Read the model definition and answer for the solid it produces. Units are mm, in the model's axes. A direction names the side the tool comes from. Coordinates: 2 decimals unless noted, no trailing zeros. Write each loop counter-clockwise with the first axis right and the second up, starting at its lowest first coordinate (ties: lowest second). Pieces come first, ordered by that corner, then holes. Notation, with made-up numbers: (33, 2.25) -> (56, 2.25) arc R14 ccw to (56, 20.25) -> close; hole circle Ø2 at (73.25, 89). An arc over 180 degrees is marked (long way). Return JSON: item names as keys, results as strings.
from build123d import *

# Parameters (mm, degrees)
BOSS_EXTRUDE1_DEPTH = 3.81
SKETCH3_R           = 2.3749
BOSS_EXTRUDE2_DEPTH = 8.89


with BuildPart() as part:
    # Sketch1 → Boss-Extrude1 (new body)
    with BuildSketch(Plane(origin=(0, 0, 0), x_dir=(-1, 0, 0), z_dir=(0, 0, 1))):
        with BuildLine():
            Line((22.628547269, -66.432139719), (24.16561852, -64.81086345))
            ThreePointArc((24.16561852, -64.81086345), (34.487993287, -48.673067402), (38.1, -29.859952573))
            Line((38.1, -29.859952573), (38.1, -15.158740079))
            Line((38.1, -15.158740079), (19.05, -15.158740079))
            Line((19.05, -15.158740079), (19.05, -38.1))
            ThreePointArc((19.05, -38.1), (15.330256121, -47.080256121), (6.35, -50.8))
            Line((6.35, -50.8), (-6.35, -50.8))
            ThreePointArc((-6.35, -50.8), (-15.330256121, -47.080256121), (-19.05, -38.1))
            Line((-19.05, -38.1), (-19.05, -15.158740079))
            Line((-19.05, -15.158740079), (-38.1, -15.158740079))
            Line((-38.1, -15.158740079), (-38.1, -29.859952521))
            ThreePointArc((-38.1, -29.859952521), (-34.48799327, -48.673067394), (-24.165618457, -64.810863465))
            Line((-24.165618457, -64.810863465), (-22.628547192, -66.432139742))
            ThreePointArc((-22.628547192, -66.432139742), (-16.748004858, -70.533761809), (-9.725580732, -71.979320912))
            Line((-9.725580732, -71.979320912), (9.725580787, -71.979320912))
            ThreePointArc((9.725580787, -71.979320912), (16.748004927, -70.533761802), (22.628547269, -66.432139719))
        make_face()
    extrude(amount=BOSS_EXTRUDE1_DEPTH)

    # Sketch3 → Boss-Extrude2 (add)
    with BuildSketch(Plane.XY):
        with Locations((-24.622521445, 58.445286133)):
            Circle(SKETCH3_R)
        with Locations((-22.865421031, 29.826745675)):
            Circle(SKETCH3_R)
    boss_extrude2 = extrude(amount=BOSS_EXTRUDE2_DEPTH)

    # Mirror1: Boss-Extrude2 across plane
    add(boss_extrude2.mirror(Plane(origin=(0, 0, 0), x_dir=(0, 0, 1), z_dir=(1, 0, 0))))


solid = part.part
1. The part is cut by section D-D (z = 6.25). Determine the outline of the cut face in (x, y), then the cut area to 3 significant figures.
Taken from the geometry:
{"outline": "circle Ø4.75 at (-24.62, 58.45); circle Ø4.75 at (-22.87, 29.83); circle Ø4.75 at (22.87, 29.83); circle Ø4.75 at (24.62, 58.45)", "area": "70.9 mm2"}
2. Consider L1, parallel to Y at x = 1.5, z = 3; L2, parallel to Z at x = -26, y = 24; L3, parallel to X at y = 21, z = 3.5. Determine where each line is inside the solid, lowest interval first.
Taken from the geometry:
{"L1": "y = 50.8 to 71.98", "L2": "z = 0 to 3.81", "L3": "x = -38.1 to -19.05, 19.05 to 38.1"}
3. The part is cut by section A-A (y = 40.5). Determine the outline of the cut face in (x, z), then the cut area to 3 significant figures.
Taken from the geometry:
{"outline": "(-36.97, 0) -> (-18.82, 0) -> (-18.82, 3.81) -> (-36.97, 3.81) -> close; (18.82, 0) -> (36.97, 0) -> (36.97, 3.81) -> (18.82, 3.81) -> close", "area": "138 mm2"}
4. For a pull along X with two mould halves and no side action, classify faces 4 (the face through (28, 15.159, 2)), 5 (the face through (-23.35, 60.45, 6.31)), 6 (the face through (-34.39, 48.92, 1.88)), 7 (the face through (34.59, 48.42, 1.88)) as +X half, -X half, draft (parallel to the pull), parting line (faces both ways), or undercut.
Taken from the geometry:
{"face 4": "draft", "face 5": "undercut", "face 6": "-X half", "face 7": "+X half"}
5. Flat-ended cylindrical pins translate along their axes: pin 1 Ø1.9 at (y, z) = (30.5, 1) entering from +X; pin 2 Ø1.1 at (x, z) = (-1.5, 2.5) entering from -Y; pin 3 Ø2 at (x, z) = (28, 4.5) entering from +Y; pin 4 Ø2 at (x, z) = (16, 4) entering from -Y. Find the tip coordinate at first contact, or state that the pin passes through.
Taken from the geometry:
{"pin 1": "stops at x = 38.1", "pin 2": "stops at y = 50.8", "pin 3": "stops at y = 61.21", "pin 4": "stops at y = 45.05"}
6. A tool of negligible diameter and unlimited length cuts with its end or side. For faces 1 (the face through (15.23, 47.18, 1.88)), 2 (the face through (-20.67, 28.92, 6.31)), 3 (the face through (0, 71.979, 2)), from which of +Z, -Z, +X, -X, +Y, -Y can it reach the whole face along a straight path? Write none if from no direction.
Taken from the geometry:
{"face 1": "+Z, -Z, -Y", "face 2": "+Z", "face 3": "+Z, -Z, +X, -X, +Y"}
7. The part is cut by section B-B (z = 2.25). Determine the outline of the cut face in (x, y).
Taken from the geometry:
{"outline": "(-38.1, 15.16) -> (-19.05, 15.16) -> (-19.05, 38.1) arc R12.7 cw to (-6.35, 50.8) -> (6.35, 50.8) arc R12.7 cw to (19.05, 38.1) -> (19.05, 15.16) -> (38.1, 15.16) -> (38.1, 29.86) arc R50.8 ccw to (24.17, 64.81) -> (22.63, 66.43) arc R17.78 ccw to (9.73, 71.98) -> (-9.73, 71.98) arc R17.78 ccw to (-22.63, 66.43) -> (-24.17, 64.81) arc R50.8 ccw to (-38.1, 29.86) -> close"}
8. The part is cut by section C-C (x = 1). Determine the outline of the cut face in (y, z), then the cut area to 3 significant figures.
Taken from the geometry:
{"outline": "(50.8, 0) -> (71.98, 0) -> (71.98, 3.81) -> (50.8, 3.81) -> close", "area": "80.7 mm2"}
